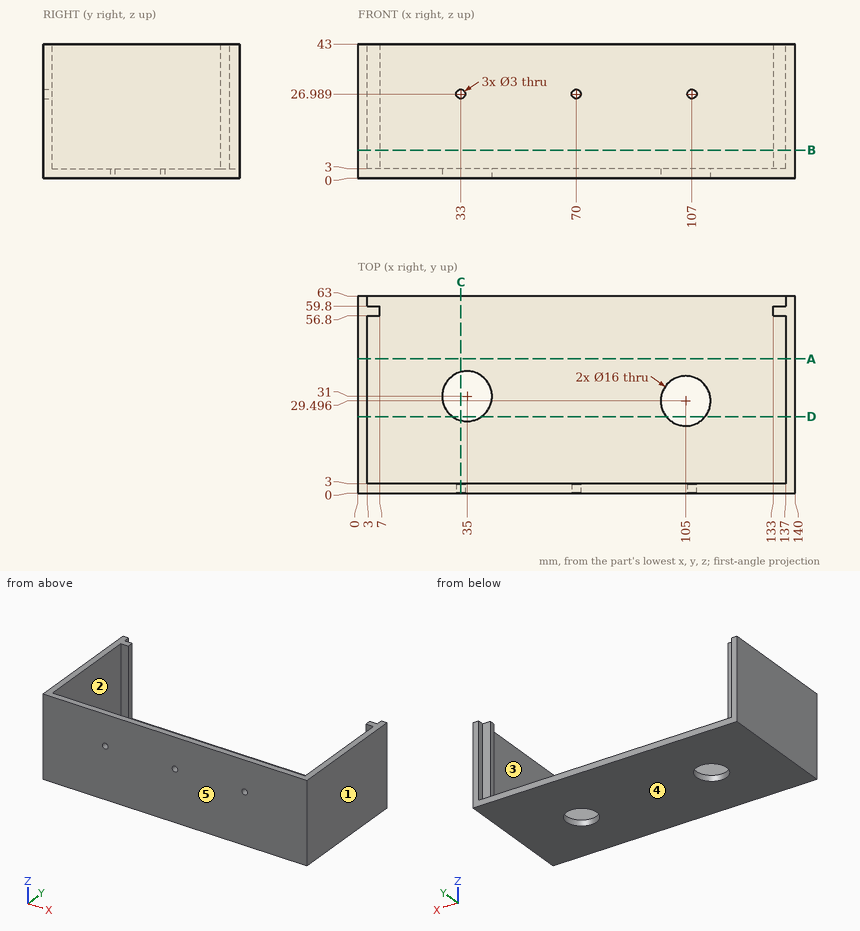
Source: three-view drawing plus pictorial views. Frame: mm from the lowest corner of the part. A direction names the side the tool comes from. Coordinates: 2 decimals unless noted, no trailing zeros. Order: outer loops, then holes, each group sorted by start corner. A loop starts at its lowest first (then second) coordinate and runs counter-clockwise, first axis right, second up. Notation, with made-up numbers: M -21,6 L -17,6 A32 ccw -17,35 Z; hole C 31,-28 d9. An arc over 180 degrees is marked long. Write each question's results on one line, items separated by ' | '. Start each with the question number.
1. Pin query (flat end, axial travel): pin 1 (12 mm diameter, centred on x = 51.5, y = 51, fed in from -Z); pin 2 (2 mm diameter, centred on x = 134, z = 21.5, fed in from +Y); pin 3 (1.5 mm diameter, centred on x = 85, z = 38.5, fed in from +Y). Return the tip coordinate at first contact, or that it passes through.
2. Material intervals for L1, parallel to X at y = 37.5, z = 15; L2, parallel to Z at x = 33, y = 2.1; L3, parallel to Z at x = 72.5, y = 27.5, sorted ascending.
3. Reachability of the marked faces 1 and 2 from +Z, -Z, +X, -X, +Y, -Y: full face, straight path, thin tool, end or side. Return the list, or none.
4. Section B-B, the plane z = 9. Return the cut outline in (x, y), then the cut area to 3 significant figures.
5. Draft query along Y for the marked faces 3, 4 and 5. Return one class per face: +Y half, -Y half, draft (parallel to the pull), parting line (faces both ways), or undercut.
6. Section D-D, the plane y = 24.5. Return the cut outline in (x, z).
7. Section A-A, the plane y = 43. Return the cut outline in (x, z), then the cut area to 3 significant figures.
8. Section C-C, the plane x = 33. Return the cut outline in (y, z).
Solution:
1) pin 1: z = 0 | pin 2: y = 59.8 | pin 3: y = 3
2) L1: 0 to 3, 137 to 140 | L2: 0 to 25.49, 28.49 to 43 | L3: 0 to 3
3) face 1: +Z, -Z, +X, +Y, -Y | face 2: +Z
4) outline: M 0,0 L 140,0 L 140,63 L 137,63 L 137,59.8 L 133,59.8 L 133,56.8 L 137,56.8 L 137,3 L 3,3 L 3,56.8 L 7,56.8 L 7,59.8 L 3,59.8 L 3,63 L 0,63 Z | area: 804 mm²
5) face 3: undercut | face 4: draft | face 5: -Y half
6) outline: M 0,0 L 30.34,0 L 30.34,3 L 3,3 L 3,43 L 0,43 Z; M 39.66,0 L 98.75,0 L 98.75,3 L 39.66,3 Z; M 111.25,0 L 140,0 L 140,43 L 137,43 L 137,3 L 111.25,3 Z
7) outline: M 0,0 L 140,0 L 140,43 L 137,43 L 137,3 L 3,3 L 3,43 L 0,43 Z | area: 660 mm²
8) outline: M 0,0 L 23.25,0 L 23.25,3 L 3,3 L 3,25.49 L 0,25.49 Z; M 0,28.49 L 3,28.49 L 3,43 L 0,43 Z; M 38.75,0 L 63,0 L 63,3 L 38.75,3 Z
